Autodesk Inventor part; units mm, degrees
ref_plane "YZ Plane" through (0, 0, 0) normal (1, 0, 0) x (0, 1, 0)
ref_plane "XZ Plane" through (0, 0, 0) normal (0, 1, 0) x (-1, 0, 0)
ref_plane "XY Plane" through (0, 0, 0) normal (0, 0, 1) x (1, 0, 0)
sketch "Sketch1" plane through (0, 0, 0) normal (0, 0, 1) x (1, 0, 0)
  line L0 (-66.3717, -23.5619) -> (-5.3717, -23.5619)
  line L1 (-5.3717, -23.5619) -> (-5.3717, -1.5619)
  line L2 (-5.3717, -1.5619) -> (43.6283, -1.5619)
  line L3 (43.6283, -1.5619) -> (43.6283, 14.4381)
  line L4 (43.6283, 14.4381) -> (-5.3717, 14.4381)
  line L5 (-5.3717, 14.4381) -> (-5.3717, 36.4381)
  line L6 (-5.3717, 36.4381) -> (-66.3717, 36.4381)
  line L7 (-66.3717, 36.4381) -> (-66.3717, 21.4381)
  line L8 (-66.3717, 21.4381) -> (-17.3717, 21.4381)
  line L9 (-17.3717, 21.4381) -> (-17.3717, -8.5619)
  line L10 (-17.3717, -8.5619) -> (-66.3717, -8.5619)
  line L11 (-66.3717, -8.5619) -> (-66.3717, -23.5619)
  point P0 (0, 0)
  dimension "d0" = 15
  dimension "d1" = 15
  dimension "d2" = 60
  dimension "d3" = 12
  dimension "d4" = 61
  dimension "d5" = 22
  dimension "d6" = 22
  dimension "d7" = 49
  dimension "d8" = 43.6283
  dimension "d9" = 1.5619
extrude "Extrusion1" add sketch "Sketch1" along normal blind 50
fillet "Fillet1" radius 25 6 edges at (43.6283, 6.4381, 50) (43.6283, 6.4381, 0) (-66.3717, 28.9381, 50) (-66.3717, -16.0619, 50) (-66.3717, 28.9381, 0) (-66.3717, -16.0619, 0)
sketch "Sketch2" plane through (-5.3717, -23.5619, 0) normal (0, -1, 0) x (1, 0, 0)
  arc A0 (-36, 50) -> (-36, 0) centre (-36, 25) ccw
  arc A1 (24, 0) -> (24, 50) centre (24, 25) ccw
  point P0 (5.3717, 0)
hole "Hole1" at (-41.3717, -23.5619, 25) at (18.6283, -23.5619, 25) direction (0, 1, 0) diameter 18 end through all
properties part number "6_16_V"
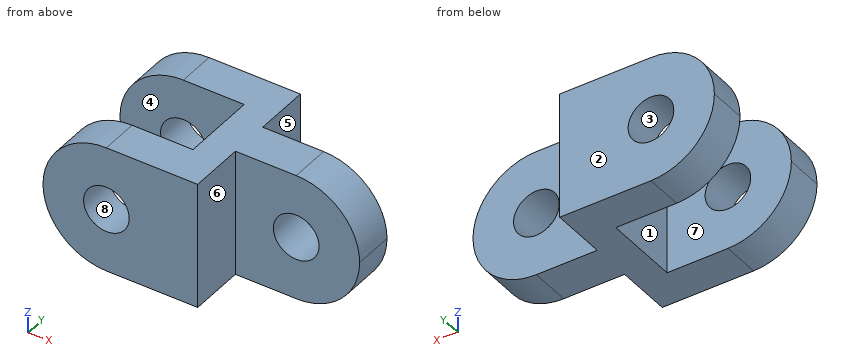
Design review of the part built by this model. Coordinates are the model's own, in mm. Face numbers are marked on the shaded views. A direction names the side the tool comes from. Give positions to 0.01 mm unless a question says otherwise; leave off trailing zeros. Order: outer loops, then holes, each group sorted by start corner. A loop starts at its lowest first (then second) coordinate and runs counter-clockwise, first axis right, second up. Notation, with made-up numbers: (68, -6.75) - (119, -6.75) arc R24 cw to (119, 9.25) - close; hole circle Ø5 at (58.5, -30). An arc over 180 degrees is marked (long way). Write item = value, one per line. Start each with the question number.
Q1. We need section D-D on y = 20. State the section outline as (x, z) points.
Q2. To check wall thickness, follow L1, parallel to X at y = -12, z = 25; L2, parallel to Y at x = -53, z = 7.5; L3, parallel to Y at x = 4, z = 41.5. State the ranges of each line that lie inside material, in increasing order. Write a range as from..to.
Q3. Mouldability with a two-part tool opening along Y and no side actions: class the marked faces 1, 2, 3 and 4 as released by +Y, released by -Y, zero draft, split by the parting line, or undercut.
Q4. We need section A-A on x = -29. State the section outline as (y, z) points.
Q5. Tool access review of the marked faces 5, 6, 7 and 8: name each direction out of +Z, -Z, +X, -X, +Y, -Y from which nothing blocks a thin tool from reaching the whole face with its end or side.
Q6. Clearance check with flat-ended pins moving along their axes: pin 1 Ø11 at (y, z) = (30, 35) entering from +X; pin 2 Ø23.5 at (x, z) = (-41.37, 25) entering from -Y; pin 3 Ø12 at (x, z) = (29.5, 19) entering from -Y; pin 4 Ø24 at (y, z) = (-11, 33) entering from +X. State where each tip first meets the part, or that it passes through.
Q7. We need section B-B on x = -48. State the section outline as (y, z) points, plus the area to 3 significant figures.
Working result:
q1.outline = (-17.37, 0) - (-5.37, 0) - (-5.37, 50) - (-17.37, 50) - close
q2.L1 = -66.37..-50.37, -32.37..-5.37
q2.L2 = -23.56..-8.56, 21.44..36.44
q2.L3 = -1.56..14.44
q3.face_1 = undercut
q3.face_2 = released by +Y
q3.face_3 = zero draft
q3.face_4 = undercut
q4.outline = (-23.56, 0) - (-8.56, 0) - (-8.56, 50) - (-23.56, 50) - close; (21.44, 0) - (36.44, 0) - (36.44, 50) - (21.44, 50) - close
q5.face_5 = +Z, -Z, +X, +Y
q5.face_6 = +Z, -Z, +X, -Y
q5.face_7 = +Z, -Z, -X
q5.face_8 = +Y, -Y
q6.pin_1 = -5.37
q6.pin_2 = -23.56
q6.pin_3 = -1.56
q6.pin_4 = 43.62
q7.outline = (-23.56, 0.89) - (-8.56, 0.89) - (-8.56, 18.91) - (-23.56, 18.91) - close; (-23.56, 31.09) - (-8.56, 31.09) - (-8.56, 49.11) - (-23.56, 49.11) - close; (21.44, 0.89) - (36.44, 0.89) - (36.44, 18.91) - (21.44, 18.91) - close; (21.44, 31.09) - (36.44, 31.09) - (36.44, 49.11) - (21.44, 49.11) - close
q7.area = 1,080 mm²
